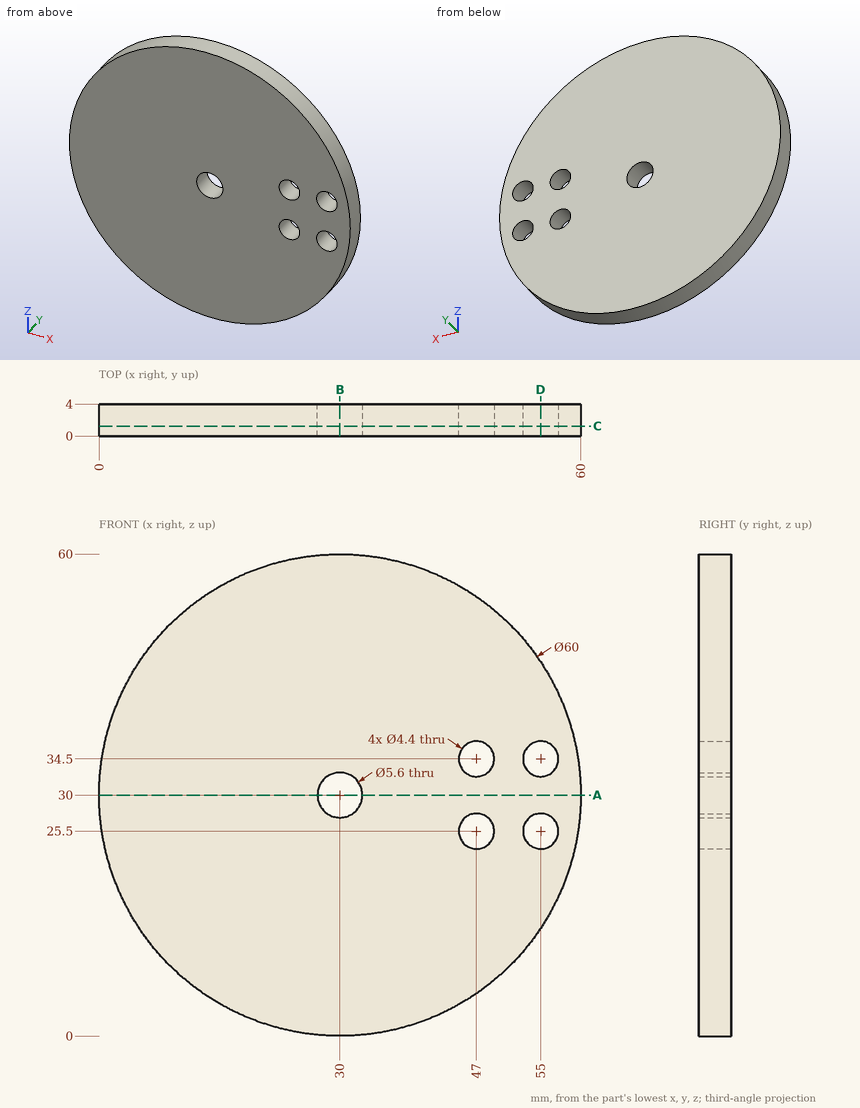
Drawing for the job (mm, zero at the part's lowest x, y, z). Round coordinates to 2 decimals unless told otherwise and drop trailing zeros. Loops run counter-clockwise (first coordinate to the right, second up) from the corner with the lowest first, then second, coordinate; pieces in that order, holes last. Notation, with made-up numbers: (79.5, 63) - (90.5, 63) arc R27 cw to (90.5, 84) - close; hole circle Ø7 at (41, 51). An arc over 180 degrees is marked (long way). Write each question's results on one line, items separated by ' | '.
(1) Saw through at C-C, the plane y = 1.25. List the corners of the cut face in (x, z), then the cut area to 3 significant figures.
Answer below:
outline: circle Ø60 at (30, 30); hole circle Ø5.6 at (30, 30); hole circle Ø4.4 at (47, 25.5); hole circle Ø4.4 at (47, 34.5); hole circle Ø4.4 at (55, 25.5); hole circle Ø4.4 at (55, 34.5) | area: 2,740 mm^2
(2) Saw through at A-A, the plane z = 30. List the corners of the cut face in (x, y).
Answer below:
outline: (0, 0) - (27.2, 0) - (27.2, 4) - (0, 4) - close; (32.8, 0) - (60, 0) - (60, 4) - (32.8, 4) - close
(3) Wall check: L1, parallel to Z at x = 30, y = 1.3; L2, parallel to Z at x = 55, y = 1.8; L3, parallel to X at y = 2.7, z = 26.5. Give the ranges that are in metal, low to high.
Answer below:
L1: z = 0 to 27.2, 32.8 to 60 | L2: z = 13.42 to 23.3, 27.7 to 32.3, 36.7 to 46.58 | L3: x = 0.2 to 45.04, 48.96 to 53.04, 56.96 to 59.8
(4) Saw through at B-B, the plane x = 30. List the corners of the cut face in (y, z).
Answer below:
outline: (0, 0) - (4, 0) - (4, 27.2) - (0, 27.2) - close; (0, 32.8) - (4, 32.8) - (4, 60) - (0, 60) - close
(5) Pin check, flat tips, straight feed: pin 1 (2 mm diameter, centred on x = 48.5, y = 2.5, fed in from -Z); pin 2 (1.5 mm diameter, centred on x = 42.5, y = 0.5, fed in from +Z). Stop position of each tip, or through.
Answer below:
pin 1: stops at z = 5.63 | pin 2: stops at z = 57.6
(6) Saw through at D-D, the plane x = 55. List the corners of the cut face in (y, z).
Answer below:
outline: (0, 13.42) - (4, 13.42) - (4, 23.3) - (0, 23.3) - close; (0, 27.7) - (4, 27.7) - (4, 32.3) - (0, 32.3) - close; (0, 36.7) - (4, 36.7) - (4, 46.58) - (0, 46.58) - close
